from build123d import *

# Parameters (mm, degrees)
F0_R     = 15
F0_R_2   = 12.5
F0_R_3   = 30
F0_R_4   = 2
F1_DEPTH = 12.7
F2_DEPTH = 40
F3_R     = 1
F4_R     = 2


with BuildPart() as f1:
    # F0 (on Top) → F1 (new body)
    with BuildSketch(Plane.XY):
        Circle(F0_R)
        Circle(F0_R_2, mode=Mode.SUBTRACT)
        Circle(F0_R_3)
        with Locations((-19.55572, -11.2905)):
            Circle(F0_R_4, mode=Mode.SUBTRACT)
        with Locations((0, -22.581)):
            Circle(F0_R_4, mode=Mode.SUBTRACT)
        with Locations((19.55572, -11.2905)):
            Circle(F0_R_4, mode=Mode.SUBTRACT)
        with Locations((-19.55572, 11.2905)):
            Circle(F0_R_4, mode=Mode.SUBTRACT)
        Circle(F0_R, mode=Mode.SUBTRACT)
        with Locations((19.55572, 11.2905)):
            Circle(F0_R_4, mode=Mode.SUBTRACT)
        with Locations((0, 22.581)):
            Circle(F0_R_4, mode=Mode.SUBTRACT)
    extrude(amount=F1_DEPTH)

    # F0 (on Top) → F2 (join)
    with BuildSketch(Plane.XY):
        Circle(F0_R)
        Circle(F0_R_2, mode=Mode.SUBTRACT)
    extrude(amount=F2_DEPTH)

    # F3
    f3_edges = [f1.edges().sort_by_distance(p)[0] for p in [
        (-15, 0, 40),
    ]]
    fillet(f3_edges, radius=F3_R)

    # F4
    f4_edges = [f1.edges().sort_by_distance(p)[0] for p in [
        (-30, 0, 12.7),
    ]]
    fillet(f4_edges, radius=F4_R)


solid = f1.part
Verification items for the finished model (mm, model axes). A direction names the side the tool comes from. Round coordinates to 2 decimals unless told otherwise and drop trailing zeros. Order: outer loops, then holes, each group sorted by start corner. A loop starts at its lowest first (then second) coordinate and runs counter-clockwise, first axis right, second up. Notation, with made-up numbers: (32, 25.5) -> (38, 25.5) arc R16 ccw to (38, 37.5) -> close; hole circle Ø9 at (47, -5). An arc over 180 degrees is marked (long way). Put each result on its own line as item: value.
1) Set-up check for faces 1 (the cylindrical face through (1.075, -20.895, 6.261)), 2 (the cylindrical face through (-14.985, 0.66, 25.666)): record each of +Z, -Z, +X, -X, +Y, -Y from which the full face is reachable in a straight line by a thin tool's end or side.
Final values:
face 1: +Z, -Z
face 2: +Z
2) Section check B-B (y = 0). Record the cut outline in (x, z).
Final values:
outline: (-30, 0) -> (-12.5, 0) -> (-12.5, 40) -> (-14, 40) arc R1 ccw to (-15, 39) -> (-15, 12.7) -> (-28, 12.7) arc R2 ccw to (-30, 10.7) -> close; (12.5, 0) -> (30, 0) -> (30, 10.7) arc R2 ccw to (28, 12.7) -> (15, 12.7) -> (15, 39) arc R1 ccw to (14, 40) -> (12.5, 40) -> close
3) Depth check by flat-ended pin: pin 1 (1.5 mm diameter, centred on x = -14.5, y = -13.5, fed in from -Z); pin 2 (10 mm diameter, centred on y = -16, z = 11, fed in from -X); pin 3 (6 mm diameter, centred on y = -16, z = 29.5, fed in from -X); pin 4 (4.5 mm diameter, centred on x = 0, y = 22.581, fed in from +Z). Enter the tip coordinate at first touch or a pass-through.
Final values:
pin 1: stops at z = 0
pin 2: stops at x = -27.91
pin 3: stops at x = -7.48
pin 4: stops at z = 12.7
4) Section check A-A (x = 0). Record the cut outline in (y, z), then the cut area to 3 significant figures.
Final values:
outline: (-30, 0) -> (-24.58, 0) -> (-24.58, 12.7) -> (-28, 12.7) arc R2 ccw to (-30, 10.7) -> close; (-20.58, 0) -> (-12.5, 0) -> (-12.5, 40) -> (-14, 40) arc R1 ccw to (-15, 39) -> (-15, 12.7) -> (-20.58, 12.7) -> close; (12.5, 0) -> (20.58, 0) -> (20.58, 12.7) -> (15, 12.7) -> (15, 39) arc R1 ccw to (14, 40) -> (12.5, 40) -> close; (24.58, 0) -> (30, 0) -> (30, 10.7) arc R2 ccw to (28, 12.7) -> (24.58, 12.7) -> close
area: 477 mm^2
5) Material ranges on line 1 (Y direction, x = 0, z = 5.5); line 2 (Z direction, x = -6, y = 15.5); line 3 (X direction, y = 9, z = 33.5), recorded low to high.
Final values:
line 1: y = -30 to -24.58, -20.58 to -12.5, 12.5 to 20.58, 24.58 to 30
line 2: z = 0 to 12.7
line 3: x = -12 to -8.67, 8.67 to 12
6) Mould release check, pull along X, two halves, no side actions. Record for faces 3 (the cylindrical face through (-29.97, 1.32, 5.28)), 4 (the cylindrical face through (18.08, -9.94, 6.26)), 5 (the flat face through (12, -12, 12.7)): +X half, -X half, draft (parallel to the pull), parting line (faces both ways), or undercut.
Final values:
face 3: parting line
face 4: undercut
face 5: draft
7) Section check D-D (z = 4). Record the cut outline in (x, y), then the cut area to 3 significant figures.
Final values:
outline: circle Ø60 at (0, 0); hole circle Ø4 at (-19.56, -11.29); hole circle Ø4 at (-19.56, 11.29); hole circle Ø25 at (0, 0); hole circle Ø4 at (0, -22.58); hole circle Ø4 at (0, 22.58); hole circle Ø4 at (19.56, -11.29); hole circle Ø4 at (19.56, 11.29)
area: 2,260 mm^2
8) Section check C-C (z = 36.5). Record the cut outline in (x, y).
Final values:
outline: circle Ø30 at (0, 0); hole circle Ø25 at (0, 0)
